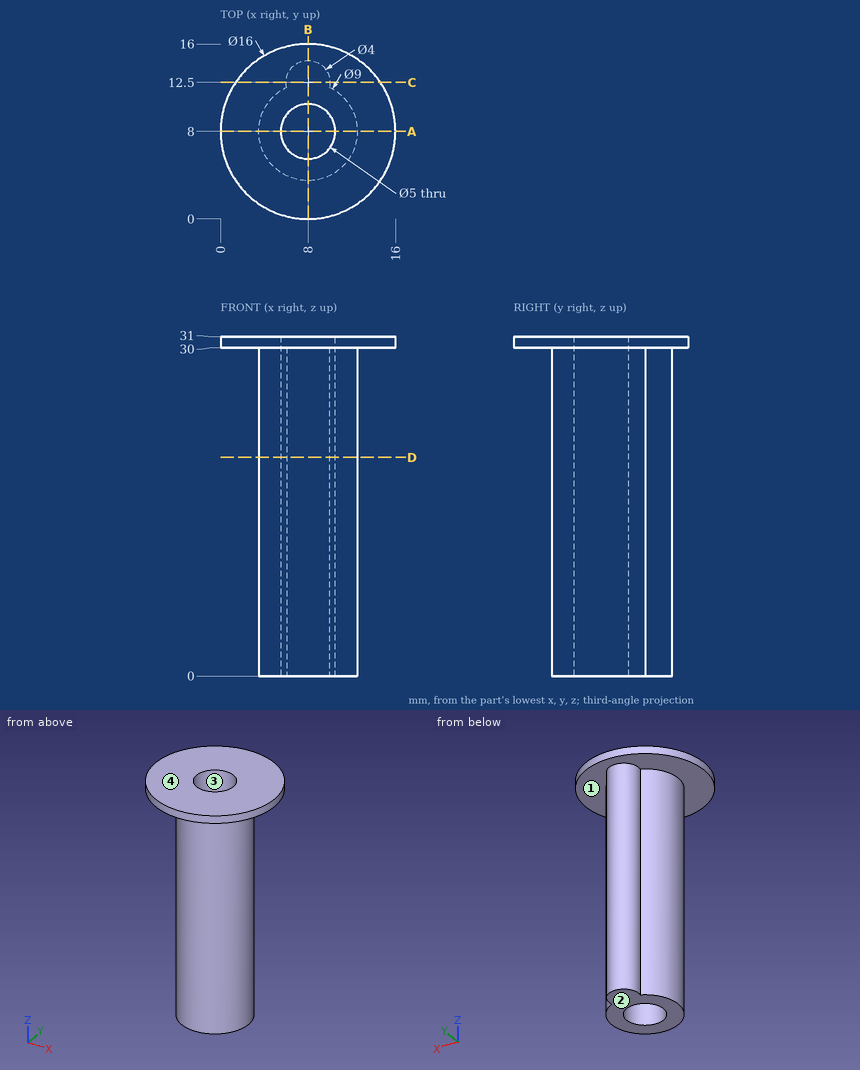
Can you work these out from the drawing? Everything is in mm from the part's minimum corner. A direction names the side the tool comes from. Coordinates: 2 decimals unless noted, no trailing zeros. Write each loop counter-clockwise with the first axis right and the second up, starting at its lowest first coordinate (ties: lowest second). Pieces come first, ordered by that corner, then holes. Notation, with made-up numbers: (29, -22.75) -> (40, -22.75) arc R16 cw to (40, -3.75) -> close; hole circle Ø10 at (79, 64.5). An arc over 180 degrees is marked (long way). Write item = value, one per line.
(1) Imagine slicing it at B-B (x = 8). Please give me the cut outline in (y, z), and give its area (3 significant figures).
Verdict:
outline = (0, 30) -> (3.5, 30) -> (3.5, 0) -> (5.5, 0) -> (5.5, 31) -> (0, 31) -> close; (10.5, 0) -> (14.5, 0) -> (14.5, 30) -> (16, 30) -> (16, 31) -> (10.5, 31) -> close
area = 191 mm^2
(2) On a 3-axis mill with a long thin cutter (end or side, diameter ignored), from which of +Z, -Z, +X, -X, +Y, -Y can I reach the whole of each face in a straight line? I mean the marked faces 1 and 2. Say none if no direction works.
Verdict:
face_1 = -Z
face_2 = -Z, +X, -X, +Y, -Y
(3) Imagine slicing it at A-A (y = 8). Please give me the cut outline in (x, z), and give its area (3 significant figures).
Verdict:
outline = (0, 30) -> (3.5, 30) -> (3.5, 0) -> (5.5, 0) -> (5.5, 31) -> (0, 31) -> close; (10.5, 0) -> (12.5, 0) -> (12.5, 30) -> (16, 30) -> (16, 31) -> (10.5, 31) -> close
area = 131 mm^2
(4) For pin 1 (1 mm diameter, centred on x = 4, y = 3.5, fed in from -Z); pin 2 (1.5 mm diameter, centred on x = 10, z = 19.5, fed in from -Y); pin 3 (6 mm diameter, centred on y = 8.5, z = 11, fed in from -X), each with a flat end and sliding along its axis, tell me the tip position at first contact or that it passes through.
Verdict:
pin_1 = 30
pin_2 = 3.68
pin_3 = 3.5
(5) Imagine slicing it at D-D (z = 20). Please give me the cut outline in (x, y).
Verdict:
outline = (6.05, 12.06) arc R4.5 ccw (long way) to (9.95, 12.06) arc R2 ccw (long way) to start; hole circle Ø5 at (8, 8)
(6) Thinking about a two-plate mould opening in Y: for the marked faces 3 and 4, which applies, +Y half, -Y half, draft (parallel to the pull), parting line (faces both ways), or undercut?
Verdict:
face_3 = undercut
face_4 = draft
(7) Imagine slicing it at C-C (y = 12.5). Please give me the cut outline in (x, z).
Verdict:
outline = (1.39, 30) -> (6, 30) -> (6, 0) -> (10, 0) -> (10, 30) -> (14.61, 30) -> (14.61, 31) -> (1.39, 31) -> close
(8) If I drill on probe 1 along Z at (x, y) = (8.25, 3); probe 2 along X at (y, z) = (7.75, 29.5); probe 3 along Y at (x, z) = (9.75, 27.5), over which ranges is the centre line in solid material (lowest first)?
Verdict:
probe_1 = 30 to 31
probe_2 = 3.51 to 5.51, 10.49 to 12.49
probe_3 = 3.85 to 6.21, 9.79 to 13.47
